Could you check a few things on this model? Use its own coordinates, in mm. Face numbers are marked on the shaded views. A direction names the side the tool comes from. Give positions to 0.01 mm unless a question says otherwise; leave off trailing zeros. Loops run counter-clockwise (first coordinate to the right, second up) from the corner with the lowest first, then second, coordinate; pieces in that order, holes last. Notation, with made-up numbers: M -8.75,26 L 11.25,26 A9 ccw 11.25,40 Z; hole C -26.75,59 d2. An arc over 180 degrees is marked long. Answer in a Markdown table with one row per item. Add a question column.
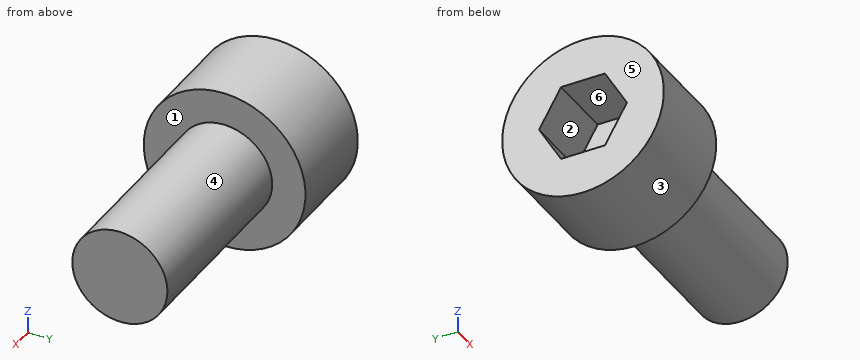
```python
from build123d import *

# Parameters (mm, degrees)
F3_DEPTH = 3.5


with BuildPart() as f1:
    # F0 (on Front) → F1 (revolve)
    with BuildSketch(Plane.XZ):
        Polygon((5, 0), (0, 0), (0, -4.25), (15, -4.25), (15, -1.75), (5, -1.75), align=None)
    revolve(axis=Axis((7.5, 0, -4.25), (-1, 0, 0)))

    # F2 (on face) → F3 (cut)
    with BuildSketch(Plane(origin=(0, 0, 0), x_dir=(0, -1, 0), z_dir=(-1, 0, 0))):
        Polygon((1.154701, -2.25), (-1.154701, -2.25), (-2.309401, -4.25), (-1.154701, -6.25), (1.154701, -6.25), (2.309401, -4.25), align=None)
    extrude(amount=-F3_DEPTH, mode=Mode.SUBTRACT)


solid = f1.part
```
Item 1: Suppose I cut it at C-C (z = -4.5). List the corners of the cut face in (x, y) for me.
Item 2: If we mould it in two halves opening along Z, with no side actions, what happens to the marked faces 4, 5 and 6? For each: +Z half, -Z half, draft (parallel to the pull), parting line (faces both ways), or undercut.
Item 3: For the marked faces 1, 2 and 3, which set-ups out of +Z, -Z, +X, -X, +Y, -Y let a thin tool reach every point of the face, with its end or its side?
Item 4: I need wall thicknesses on L1, parallel to X at y = -1, z = -7; L2, parallel to Z at x = 5.5, y = 1.5; L3, parallel to X at y = -1.25, z = -4.5. Which ranges of each line are inside material? Lowest first, please.
Item 5: Suppose I cut it at D-D (x = 6). List the corners of the cut face in (y, z) for me.
Item 6: Suppose I cut it at B-B (x = 2.5). List the corners of the cut face in (y, z) for me.
Item 7: For P1, Ø1.2, axis at y = 0.5, z = -4, coming from the -X side, with a flat end and sliding along its axis, tell me the tip position at first contact or that it passes through.
Item 8: Suppose I cut it at A-A (y = 0). List the corners of the cut face in (x, z) for me, then the cut area to 3 significant figures.
Values found:
| question | item | result |
|---|---|---|
| 1 | outline | M 0,-4.24 L 5,-4.24 L 5,-2.49 L 15,-2.49 L 15,2.49 L 5,2.49 L 5,4.24 L 0,4.24 L 0,2.17 L 3.5,2.17 L 3.5,-2.17 L 0,-2.17 Z |
| 2 | face 4 | parting line |
| 2 | face 5 | draft |
| 2 | face 6 | undercut |
| 3 | face 1 | +X |
| 3 | face 2 | -X |
| 3 | face 3 | +X, -X |
| 4 | L1 | 0 to 5 |
| 4 | L2 | -6.25 to -2.25 |
| 4 | L3 | 3.5 to 15 |
| 5 | outline | C 0,-4.25 d5 |
| 6 | outline | C 0,-4.25 d8.5; hole M -2.31,-4.25 L -1.15,-6.25 L 1.15,-6.25 L 2.31,-4.25 L 1.15,-2.25 L -1.15,-2.25 Z |
| 7 | P1 | x = 3.5 |
| 8 | outline | M 0,-8.5 L 5,-8.5 L 5,-6.75 L 15,-6.75 L 15,-1.75 L 5,-1.75 L 5,0 L 0,0 L 0,-2.25 L 3.5,-2.25 L 3.5,-6.25 L 0,-6.25 Z |
| 8 | area | 78.5 mm² |
